The listing builds one solid part. Answer for the finished solid, in the listing's coordinates (mm). Round coordinates to 2 decimals unless told otherwise and drop trailing zeros. Write each loop counter-clockwise with the first axis right and the second up, starting at its lowest first coordinate (ties: lowest second). Pieces come first, ordered by that corner, then holes.
Autodesk Inventor part; units mm, degrees
ref_plane "YZ Plane" through (0, 0, 0) normal (1, 0, 0) x (0, 1, 0)
ref_plane "XZ Plane" through (0, 0, 0) normal (0, 1, 0) x (-1, 0, 0)
ref_plane "XY Plane" through (0, 0, 0) normal (0, 0, 1) x (1, 0, 0)
sketch "スケッチ1" plane through (0, 0, 0) normal (0, 0, 1) x (1, 0, 0)
  line L0 (0, 0) -> (350, 0)
  line L1 (350, 0) -> (350, 140)
  line L2 (350, 140) -> (0, 140)
  circle A0 centre (70, 60) radius 46
  circle A1 centre (280, 60) radius 46
  line L3 (0, 140) -> (0, 0)
  line L4 (70, 60) -> (70, 156.3161)
  line L5 (280, 60) -> (280, 147.5689)
  line L6 (70, 60) -> (45.2011, 119.8698)
  line L7 (280, 60) -> (258.2896, 112.4136)
  circle A2 centre (52.3966, 102.4985) radius 1.5
  circle A3 centre (262.3966, 102.4985) radius 1.5
  circle A4 centre (27.5015, 77.6034) radius 1.5
  circle A5 centre (27.5015, 42.3966) radius 1.5
  circle A6 centre (52.3966, 17.5015) radius 1.5
  circle A7 centre (87.6034, 17.5015) radius 1.5
  circle A8 centre (112.4985, 42.3966) radius 1.5
  circle A9 centre (112.4985, 77.6034) radius 1.5
  circle A10 centre (87.6034, 102.4985) radius 1.5
  circle A11 centre (237.5015, 77.6034) radius 1.5
  circle A12 centre (237.5015, 42.3966) radius 1.5
  circle A13 centre (262.3966, 17.5015) radius 1.5
  circle A14 centre (297.6034, 17.5015) radius 1.5
  circle A15 centre (322.4985, 42.3966) radius 1.5
  circle A16 centre (322.4985, 77.6034) radius 1.5
  circle A17 centre (297.6034, 102.4985) radius 1.5
  circle A18 centre (70, 60) radius 30
  circle A19 centre (280, 60) radius 30
  dimension "d5" = 92
  dimension "d6" = 92
  dimension "d0" = 350
  dimension "d1" = 140
  dimension "d2" = 60
  dimension "d3" = 60
  dimension "d9" = 70
  dimension "d10" = 70
  dimension "d11" = 22.5
  dimension "d12" = 22.5
  dimension "d13" = 3
  dimension "d14" = 3
  dimension "d17" = 360
  dimension "d21" = 360
  dimension "d23" = 60
  dimension "d24" = 60
extrude "押し出し1" add sketch "スケッチ1" along normal blind 5 contours A1 A17 A16 A15 A14 A13 A12 A11 A3 L7 A19 L5 | L5 A19 L7 A3 A1 | A0 A10 A9 A8 A7 A6 A5 A4 A2 L6 A18 L4 | L4 A18 L6 A2 A0 | L3 L2 L1 L0
fillet "フィレット2" radius 50 2 edges at (350, 0, 2.5) (0, 0, 2.5)
equation "\"d6\" = d5"
equation "\"d2\" = d3"
equation "\"d10\" = d9"
properties part number "b_right-wr2left-wr__legparts_09(six)"
1. Section C-C on z = 3.25 is taken. Give the number of separate pieces and of enclosed holes in the cut face, plus the area to 3 significant figures.
Geometry says:
separate pieces: 1
enclosed holes: 18
area: 42,200 mm2
2. Section D-D on y = 60 is taken. Determine the outline of the cut face in (x, z), plus the area to 3 significant figures.
Geometry says:
outline: (0, 0) - (40, 0) - (40, 5) - (0, 5) - close; (100, 0) - (250, 0) - (250, 5) - (100, 5) - close; (310, 0) - (350, 0) - (350, 5) - (310, 5) - close
area: 1,150 mm2
3. Section B-B on x = 70 is taken. Determine the outline of the cut face in (y, z).
Geometry says:
outline: (0, 0) - (30, 0) - (30, 5) - (0, 5) - close; (90, 0) - (140, 0) - (140, 5) - (90, 5) - close
4. For a pull along Y with two mould halves and no side action, classify faces 1 (the face through (40.03, 58.68, 2.46)), 2 (the face through (173, 71, 0)), 3 (the face through (334.964, 14.258, 2.535)) as released by +Y, released by -Y, zero draft, split by the parting line, or undercut.
Geometry says:
face 1: undercut
face 2: zero draft
face 3: released by -Y
5. Straight lines are drawn through the part: line 1 along X through (y, z) = (16.5, 1.35); line 2 along X through (y, z) = (75, 2.9); line 3 along X through (y, z) = (50.5, 2.35). For each, find the intervals that lie inside material, in ascending order.
Geometry says:
line 1: x = 12.88 to 51.28, 53.51 to 86.49, 88.72 to 261.28, 263.51 to 296.49, 298.72 to 337.12
line 2: x = 0 to 44.02, 95.98 to 254.02, 305.98 to 350
line 3: x = 0 to 41.54, 98.46 to 251.54, 308.46 to 350
6. Section A-A on y = 36 is taken. Determine the outline of the cut face in (x, z).
Geometry says:
outline: (2, 0) - (52, 0) - (52, 5) - (2, 5) - close; (88, 0) - (262, 0) - (262, 5) - (88, 5) - close; (298, 0) - (348, 0) - (348, 5) - (298, 5) - close
